Autodesk Fusion 360 part; units mm, degrees
sketch "Skizze1" plane through (0, 0, 0) normal (0, 1, 0) x (1, 0, 0)
  line L0 (0, 0) -> (140, 0)
  line L1 (140, 0) -> (140, -46)
  line L2 (140, -46) -> (0, -46)
  line L3 (0, -46) -> (0, 0)
  circle A0 centre (4, -42) radius 1.6
  circle A1 centre (4, -4) radius 1.6
  circle A2 centre (136, -42) radius 1.6
  circle A3 centre (136, -4) radius 1.6
  line L4 (10, -36.5) -> (130, -36.5)
  line L5 (130, -36.5) -> (130, -9.5)
  line L6 (130, -9.5) -> (10, -9.5)
  line L7 (10, -9.5) -> (10, -36.5)
  line L8 (11, -36.65) -> (62.2, -36.65)
  line L9 (62.2, -36.65) -> (62.2, -9.35)
  line L10 (62.2, -9.35) -> (11, -9.35)
  line L11 (11, -9.35) -> (11, -36.65)
  line L12 (77.8, -36.65) -> (129, -36.65)
  line L13 (129, -36.65) -> (129, -9.35)
  line L14 (129, -9.35) -> (77.8, -9.35)
  line L15 (77.8, -9.35) -> (77.8, -36.65)
  circle A4 centre (13.8, -33.85) radius 1.05
  circle A5 centre (59.4, -33.85) radius 1.05
  circle A6 centre (13.8, -12.15) radius 1.05
  circle A7 centre (59.4, -12.15) radius 1.05
  circle A8 centre (80.6, -33.85) radius 1.05
  circle A9 centre (80.6, -12.15) radius 1.05
  circle A10 centre (126.2, -33.85) radius 1.05
  circle A11 centre (126.2, -12.15) radius 1.05
  line L16 (8, -31.1) -> (132, -31.1)
  line L17 (132, -31.1) -> (132, -15.1)
  line L18 (132, -15.1) -> (8, -15.1)
  line L19 (8, -15.1) -> (8, -31.1)
  circle A12 centre (7, -36) radius 1.6
  circle A13 centre (133, -10) radius 1.6
  circle A14 centre (133, -36) radius 1.6
  circle A15 centre (7, -10) radius 1.6
  dimension "d1" = 140
  dimension "d2" = 46
  dimension "d3" = 3.2
  dimension "d4" = 3.2
  dimension "d5" = 3.2
  dimension "d6" = 3.2
  dimension "d7" = 132
  dimension "d8" = 38
  dimension "d9" = 38
  dimension "d10" = 132
  dimension "d11" = 4
  dimension "d12" = 4
  dimension "d60" = 120
  dimension "d61" = 27
  dimension "d62" = 9.5
  dimension "d63" = 10
  dimension "d64" = 1
  dimension "d65" = 1
  dimension "d66" = 51.2
  dimension "d67" = 51.2
  dimension "d68" = 27.3
  dimension "d69" = 27.3
  dimension "d70" = 0.15
  dimension "d71" = 0.15
  dimension "d72" = 2.1
  dimension "d73" = 2.1
  dimension "d74" = 2.1
  dimension "d75" = 2.1
  dimension "d76" = 2.1
  dimension "d77" = 2.1
  dimension "d78" = 2.1
  dimension "d79" = 2.1
  dimension "d80" = 2.8
  dimension "d81" = 2.8
  dimension "d82" = 2.8
  dimension "d83" = 2.8
  dimension "d84" = 45.6
  dimension "d85" = 45.6
  dimension "d86" = 21.7
  dimension "d87" = 21.7
  dimension "d88" = 45.6
  dimension "d89" = 21.7
  dimension "d90" = 21.7
  dimension "d91" = 16
  dimension "d92" = 124
  dimension "d95" = 5.55
  dimension "d115" = 3.2
  dimension "d116" = 3.2
  dimension "d117" = 3.2
  dimension "d118" = 3.2
  dimension "d121" = 126
  dimension "d123" = 10
  dimension "d124" = 7
  dimension "d125" = 26
  dimension "d126" = 126
  dimension "d127" = 26
  dimension "d128" = 36
  dimension "d129" = 133
  dimension "d130" = 133
  dimension "d131" = 8
extrude "Extrusion1" add sketch "Skizze1" along normal blind 3 contours L0 L1 L2 L3 | L4 L7 L11 L16 | L4 L9 L11 L16 | L4 L8 L9 L11 | L7 L16 L18 L19 | L7 L11 L16 L18 | L4 L9 L15 L16 | L9 L11 L16 L18 | L6 L7 L11 L18 | L4 L13 L15 L16 | L4 L12 L13 L15 | L9 L15 L16 L18 | L6 L9 L11 L18 | L4 L5 L13 L16 | L13 L15 L16 L18 | L6 L9 L15 L18 | L6 L9 L10 L11 | L5 L13 L16 L18 | L6 L13 L15 L18 | L5 L16 L17 L18 | L5 L6 L13 L18 | L6 L13 L14 L15 | A4 | A5 | A6 | A7 | A8 | A9 | A10 | A11 | A12 | A13 | A14 | A15
sketch "Skizze4" plane through (0, 0, 0) normal (0, 1, 0) x (1, 0, 0)
  line L0 (7, -39) -> (133, -39)
  line L1 (133, -33) -> (133, -13)
  line L2 (133, -7) -> (7, -7)
  line L3 (7, -13) -> (7, -33)
  arc A0 (7, -33) -> (7, -39) centre (7, -36) ccw
  arc A1 (133, -13) -> (133, -7) centre (133, -10) ccw
  arc A2 (133, -39) -> (133, -33) centre (133, -36) ccw
  arc A3 (7, -7) -> (7, -13) centre (7, -10) ccw
  circle A4 centre (7, -36) radius 1.6
  circle A5 centre (7, -10) radius 1.6
  circle A6 centre (133, -36) radius 1.6
  circle A7 centre (133, -10) radius 1.6
  dimension "d99" = 126
  dimension "d100" = 32
  dimension "d101" = 6
  dimension "d102" = 3
  dimension "d103" = 6
  dimension "d104" = 6
  dimension "d105" = 6
  dimension "d106" = 3
  dimension "d107" = 3
  dimension "d108" = 3
  dimension "d109" = 7
  dimension "d110" = 7
  dimension "d111" = 3.2
  dimension "d112" = 3.2
  dimension "d113" = 3.2
  dimension "d114" = 3.2
sketch "Skizze5" plane through (0, 0, 0) normal (0, 1, 0) x (1, 0, 0)
  line L0 (7, -39) -> (133, -39)
  arc A0 (7, -33) -> (7, -39) centre (7, -36) ccw
  line L1 (7, -13) -> (7, -33)
  arc A1 (7, -7) -> (7, -13) centre (7, -10) ccw
  line L2 (133, -7) -> (7, -7)
  arc A2 (133, -13) -> (133, -7) centre (133, -10) ccw
  line L3 (133, -33) -> (133, -13)
  arc A3 (133, -39) -> (133, -33) centre (133, -36) ccw
  line L4 (77.8, -9.35) -> (77.8, -36.65)
  line L5 (77.8, -36.65) -> (129, -36.65)
  line L6 (129, -36.65) -> (129, -9.35)
  line L7 (129, -9.35) -> (77.8, -9.35)
  line L8 (62.2, -9.35) -> (11, -9.35)
  line L9 (62.2, -36.65) -> (62.2, -9.35)
  line L10 (11, -9.35) -> (11, -36.65)
  line L11 (11, -36.65) -> (62.2, -36.65)
  line L12 (17.25, -34.35) -> (59.97, -34.35)
  line L13 (59.97, -34.35) -> (59.97, -11.65)
  line L14 (59.97, -11.65) -> (17.25, -11.65)
  line L15 (17.25, -11.65) -> (17.25, -34.35)
  line L16 (122.75, -34.35) -> (80.03, -34.35)
  line L17 (80.03, -34.35) -> (80.03, -11.65)
  line L18 (80.03, -11.65) -> (122.75, -11.65)
  line L19 (122.75, -11.65) -> (122.75, -34.35)
  dimension "d132" = 126
  dimension "d133" = 32
  dimension "d134" = 6
  dimension "d135" = 3
  dimension "d136" = 6
  dimension "d137" = 6
  dimension "d138" = 6
  dimension "d139" = 3
  dimension "d140" = 3
  dimension "d141" = 3
  dimension "d142" = 51.2
  dimension "d143" = 51.2
  dimension "d144" = 27.3
  dimension "d145" = 27.3
  dimension "d146" = 7
  dimension "d147" = 7
  dimension "d148" = 9.35
  dimension "d149" = 9.35
  dimension "d150" = 11
  dimension "d151" = 77.8
  dimension "d152" = 6.25
  dimension "d153" = 6.25
  dimension "d154" = 2.23
  dimension "d155" = 2.23
  dimension "d156" = 2.3
  dimension "d157" = 2.3
  dimension "d158" = 2.3
  dimension "d159" = 2.3
sketch "Skizze6" plane through (0, 0, 0) normal (0, 1, 0) x (1, 0, 0)
  line L0 (4, 0) -> (211, 0)
  line L1 (215, -4) -> (215, -58)
  line L2 (211, -62) -> (4, -62)
  line L3 (0, -58) -> (0, -4)
  circle A0 centre (10.75, -53) radius 2.25
  circle A1 centre (10.75, -9) radius 2.25
  circle A2 centre (204.25, -53) radius 2.25
  circle A3 centre (204.25, -9) radius 2.25
  arc A4 (0, -58) -> (4, -62) centre (4, -58) ccw
  arc A5 (4, 0) -> (0, -4) centre (4, -4) ccw
  arc A6 (211, -62) -> (215, -58) centre (211, -58) ccw
  arc A7 (215, -4) -> (211, 0) centre (211, -4) ccw
  point P0 (215, 0)
  point P1 (0, -62)
  dimension "d160" = 62
  dimension "d161" = 215
  dimension "d162" = 4.5
  dimension "d163" = 4.5
  dimension "d164" = 4.5
  dimension "d165" = 4.5
  dimension "d167" = 193.5
  dimension "d168" = 44
  dimension "d170" = 9
  dimension "d171" = 10.75
  dimension "d172" = 4
  dimension "d173" = 4
  dimension "d174" = 4
  dimension "d175" = 4
Here's how the part is built. I have some questions about the finished solid (model axes, mm). Give positions to 0.01 mm unless a question says otherwise; leave off trailing zeros. Write each loop counter-clockwise with the first axis right and the second up, starting at its lowest first coordinate (ties: lowest second). Pieces come first, ordered by that corner, then holes.
(1) Imagine slicing it at B-B, the plane x = 4. Write out the boundary of the cut face in (y, z).
Output values:
outline: (0, 0) - (3, 0) - (3, 2.4) - (0, 2.4) - close; (0, 5.6) - (3, 5.6) - (3, 40.4) - (0, 40.4) - close; (0, 43.6) - (3, 43.6) - (3, 46) - (0, 46) - close
(2) Imagine slicing it at A-A, the plane z = 42. Write out the boundary of the cut face in (x, y).
Output values:
outline: (0, 0) - (2.4, 0) - (2.4, 3) - (0, 3) - close; (5.6, 0) - (134.4, 0) - (134.4, 3) - (5.6, 3) - close; (137.6, 0) - (140, 0) - (140, 3) - (137.6, 3) - close
(3) Will this pin go through, and if not, where does the flat tip stop? pin 1 (5 mm diameter, centred on x = 54, z = 15, fed in from -Y).
Output values:
pin 1: stops at y = 0
(4) If I drill on L1, parallel to X at y = 0.65, z = 42; L2, parallel to Z at x = 4, y = 1.2; L3, parallel to X at y = 0.9, z = 3, over which ranges is the centre line in solid material (lowest first)?
Output values:
L1: x = 0 to 2.4, 5.6 to 134.4, 137.6 to 140
L2: z = 0 to 2.4, 5.6 to 40.4, 43.6 to 46
L3: x = 0 to 2.75, 5.25 to 134.75, 137.25 to 140
(5) Thinking about a two-plate mould opening in Z: for faces 1 (the face through (71, 1, 46)), 2 (the face through (0, 1, 23)), 3 (the face through (137.48, 1.48, 3.39)), which applies, pulls with the +Z half, pulls with the -Z half, needs draft (parallel to the pull), parting line crosses it, or undercut?
Output values:
face 1: pulls with the +Z half
face 2: needs draft
face 3: undercut
